The model under review builds one solid part; all positions refer to its coordinate system, in mm. A direction names the side the tool comes from. Give positions to 0.01 mm unless a question says otherwise; leave off trailing zeros. Loops run counter-clockwise (first coordinate to the right, second up) from the corner with the lowest first, then second, coordinate; pieces in that order, holes last. Notation, with made-up numbers: (38, -2.5) - (43, -2.5) arc R13 ccw to (43, 18.5) - close; hole circle Ø8 at (-9.75, 18). An arc over 180 degrees is marked (long way). Return JSON: item names as keys, results as strings. Group by question number.
```python
from build123d import *

# Parameters (mm, degrees)
F1_DEPTH = 25.4
F3_DEPTH = 25.2600312233


with BuildPart() as f1:
    # F0 (on Front) → F1 (new body)
    with BuildSketch(Plane.XZ):
        Polygon((28.8711190224, 19.7296105325), (28.8711190224, 62.7946555614), (-28.8711190224, 62.7946555614), (-28.8711190224, -21.6803327203), (-28.8711190224, -35.6886684895), (28.8711190224, -35.6886684895), align=None)
        with BuildLine():
            Line((-28.8711190224, 62.7946555614), (28.8711190224, 62.7946555614))
            ThreePointArc((28.8711190224, 62.7946555614), (27.4521603023, 71.7344770551), (23.3347622032, 79.7955492593))
            ThreePointArc((23.3347622032, 79.7955492593), (-8.9398214937, 90.2468158638), (-28.8711190224, 62.7946555614))
        make_face()
        with BuildLine():
            ThreePointArc((23.3347622032, 79.7955492593), (27.4521603023, 71.7344770551), (28.8711190224, 62.7946555614))
            Line((28.8711190224, 62.7946555614), (62.2528098973, 64.1079097986))
            Line((62.2528098973, 64.1079097986), (62.2528098973, 79.7955492593))
            Line((62.2528098973, 79.7955492593), (23.3347622032, 79.7955492593))
        make_face()
        Polygon((74.5094120502, 19.7296105325), (28.8711190224, 19.7296105325), (28.8711190224, -35.6886684895), (89.7200107574, -35.6886684895), (89.7200107574, -23.3990810812), (74.8348683119, -23.3990810812), (74.8348683119, -10.4444716126), (89.7200107574, -10.4444716126), (89.7200107574, 0), (74.8348683119, 0), (74.8348683119, 6.5229041502), (89.7200107574, 6.5229041502), (89.7200107574, 19.7296105325), align=None)
        Polygon((-28.8711190224, -35.6886684895), (-28.8711190224, -21.6803327203), (-42.6678210497, 23.781247437), (-62.8544837236, -15.207156539), (-49.6445633471, -15.207156539), (-49.6445633471, -25.6738718599), (-59.5784634352, -25.6738718599), (-59.5784634352, -35.6886684895), align=None)
        Polygon((28.8711190224, -62.7946555614), (28.8711190224, -35.6886684895), (-28.8711190224, -35.6886684895), (-28.8711190224, -62.7946555614), (-16.2400081754, -62.7946555614), (12.0457587764, -62.7946555614), align=None)
        Polygon((19.5835158229, -118.1614845991), (28.8711190224, -62.7946555614), (12.0457587764, -62.7946555614), (12.0457587764, -126.8014013767), (28.8711190224, -126.8014013767), align=None)
        Polygon((-16.2400081754, -62.7946555614), (-28.8711190224, -62.7946555614), (-28.8711190224, -115.8453673124), (-19.3075612187, -121.8000352383), align=None)
        Polygon((-19.3075612187, -121.8000352383), (-28.8711190224, -115.8453673124), (-28.8711190224, -127.7547031641), (-9.7440034151, -127.7547031641), align=None)
    extrude(amount=F1_DEPTH)

    # F2 (on face) → F3 (join)
    with BuildSketch(Plane(origin=(0, 0, 0), x_dir=(-1, 0, 0), z_dir=(0, 1, 0))):
        with BuildLine():
            ThreePointArc((28.8711190224, -61.7056259644), (124.1382439979, -10.8280309146), (162.1938628718, 90.2468158638))
            ThreePointArc((162.1938628718, 90.2468158638), (-55.7393219165, 229.1835266585), (-89.7200107575, -27.0265344717))
            Line((-89.7200107574, -27.0265344717), (-89.7200107574, -23.3990810812))
            Line((-89.7200107574, -23.3990810812), (-74.8348683119, -23.3990810812))
            Line((-74.8348683119, -23.3990810812), (-74.8348683119, -10.4444716126))
            Line((-74.8348683119, -10.4444716126), (-89.7200107574, -10.4444716126))
            Line((-89.7200107574, -10.4444716126), (-89.7200107574, 0))
            Line((-89.7200107574, 0), (-74.8348683119, 0))
            Line((-74.8348683119, 0), (-74.8348683119, 6.5229041502))
            Line((-74.8348683119, 6.5229041502), (-89.7200107574, 6.5229041502))
            Line((-89.7200107574, 6.5229041502), (-89.7200107574, 19.7296105325))
            Line((-89.7200107574, 19.7296105325), (-28.8711190224, 19.7296105325))
            Line((-28.8711190224, 19.7296105325), (-28.8711190224, 62.7946555614))
            Line((-28.8711190224, 62.7946555614), (-62.2528098973, 64.1079097986))
            Line((-62.2528098973, 64.1079097986), (-62.2528098973, 79.7955492593))
            Line((-62.2528098973, 79.7955492593), (-23.3347622032, 79.7955492593))
            ThreePointArc((-23.3347622032, 79.7955492593), (8.9398214937, 90.2468158638), (28.8711190224, 62.7946555614))
            Line((28.8711190224, 62.7946555614), (28.8711190224, -21.6803327203))
            Line((28.8711190224, -21.6803327203), (42.6678210497, 23.781247437))
            Line((42.6678210497, 23.781247437), (62.8544837236, -15.207156539))
            Line((62.8544837236, -15.207156539), (49.6445633471, -15.207156539))
            Line((49.6445633471, -15.207156539), (49.6445633471, -25.6738718599))
            Line((49.6445633471, -25.6738718599), (59.5784634352, -25.6738718599))
            Line((59.5784634352, -25.6738718599), (59.5784634352, -35.6886684895))
            Line((59.5784634352, -35.6886684895), (28.8711190224, -35.6886684895))
            Line((28.8711190224, -35.6886684895), (28.8711190224, -61.7056259644))
        make_face()
    extrude(amount=-F3_DEPTH)


solid = f1.part
```
1) We need section C-C, the plane x = -131. Write out the cut boundary in (y, z), plus the area to 3 significant figures.
2) Draft analysis for pull direction Z (two halves, no side actions). For faces 1 (the face through (89.72, -13, -32)), 2 (the face through (20, -13, -126.801)), 3 (the face through (-14.46, -12.52, -124.82)), 4 (the face through (24.29, -12.52, -122.54)), state which applies: +Z half, -Z half, draft (parallel to the pull), parting line (faces both ways), or undercut.
3) We need section A-A, the plane y = -13.5. Write out the cut boundary in (x, z).
4) To check wall thickness, follow line 1 (Y direction, x = -100, z = 74); line 2 (Z direction, x = -11.5, y = -16.75); line 3 (X direction, y = -8.25, z = 74). State the ranges of each line that lie inside material, in increasing order.
5) Tool access review of faces 5 (the face through (12.046, -13, -94)), 6 (the face through (-2, -13, -62.795)), 7 (the face through (59, -13, -35.689)): name each direction out of +Z, -Z, +X, -X, +Y, -Y from which nothing blocks a thin tool from reaching the whole face with its end or side.
6) For pin 1 Ø10 at (y, z) = (-18, 20) entering from -X; pin 2 Ø6 at (y, z) = (-15, -68.5) entering from +X; pin 3 Ø1.5 at (x, y) = (54.5, -20.5) entering from -Z, all flat-tipped, find the tip position at first contact; note any pin that passes through.
7) We need section B-B, the plane z = 166. Write out the cut boundary in (x, y), plus the area to 3 significant figures.
Findings:
{
 "1": {"outline": "(-25.26, -2.43) - (0, -2.43) - (0, 182.92) - (-25.26, 182.92) - close", "area": "4,680 mm^2"},
 "2": {"face 1": "draft", "face 2": "-Z half", "face 3": "undercut", "face 4": "undercut"},
 "3": {"outline": "(-28.87, -127.75) - (-9.74, -127.75) - (-19.31, -121.8) - (-16.24, -62.79) - (12.05, -62.79) - (12.05, -126.8) - (28.87, -126.8) - (19.58, -118.16) - (28.87, -62.79) - (28.87, -35.69) - (89.72, -35.69) - (89.72, -27.03) arc R153.25 ccw (long way) to (-28.87, -61.71) - close"},
 "4": {"line 1": "y = -25.26 to 0", "line 2": "z = -127.75 to -126.66, -62.79 to 243.48", "line 3": "x = -161.33 to 143.45"},
 "5": {"face 5": "-Z, +Y, -Y", "face 6": "+Y, -Y", "face 7": "-Z, +X, +Y, -Y"},
 "6": {"pin 1": "stops at x = -147.61", "pin 2": "stops at x = 28.42", "pin 3": "stops at z = -35.69"},
 "7": {"outline": "(-142.16, -25.26) - (124.28, -25.26) - (124.28, 0) - (-142.16, 0) - close", "area": "6,730 mm^2"}
}
